Geometry check sheet. Reference: drawing and pictorial views, mm from the part's lowest x, y, z. A direction names the side the tool comes from. Give positions to 0.01 mm unless a question says otherwise; leave off trailing zeros. Write each loop counter-clockwise with the first axis right and the second up, starting at its lowest first coordinate (ties: lowest second). Pieces come first, ordered by that corner, then holes. Notation, with made-up numbers: M 82,47.25 L 104,47.25 A20 cw 104,83.25 Z; hole C -13.5,10 d4. An arc over 180 degrees is marked long. Answer as a JSON object with one key per item and string values.
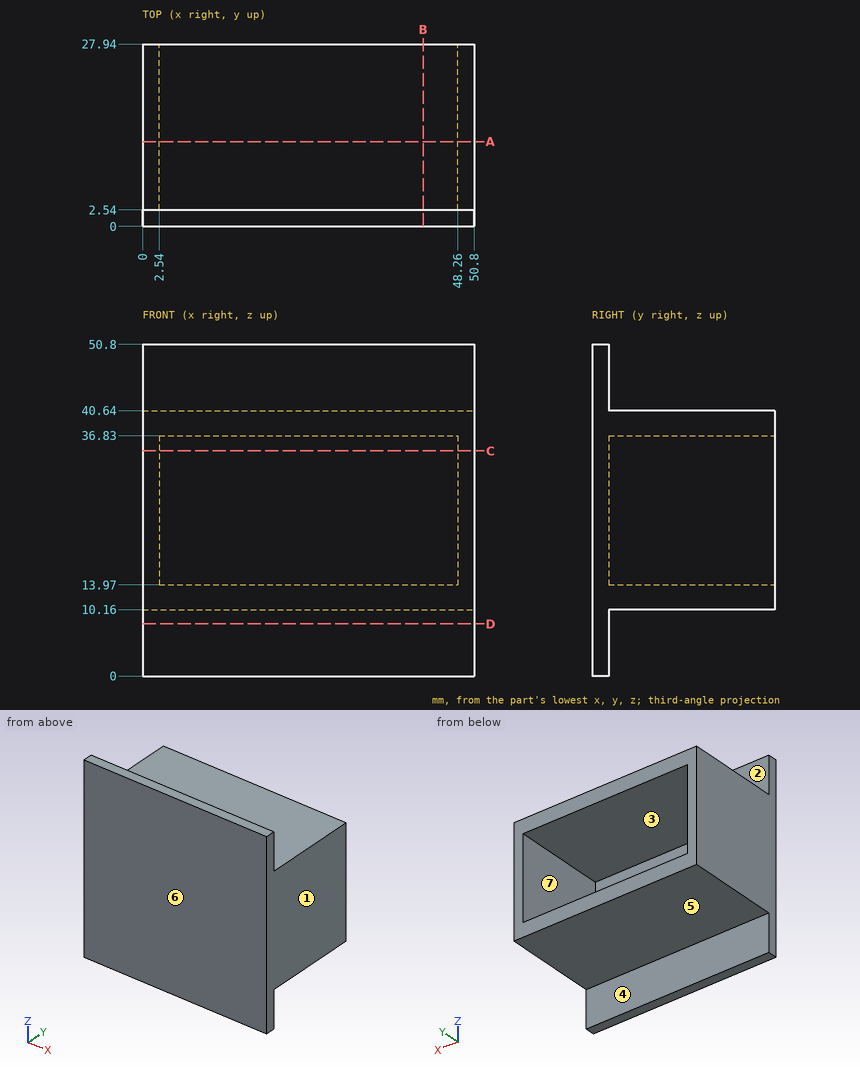
1) Release check for a two-part mould opening along Z. For the marked faces 5, 6 and 7 record: pulls with the +Z half, pulls with the -Z half, needs draft (parallel to the pull), parting line crosses it, or undercut.
Completed:
{"face 5": "pulls with the -Z half", "face 6": "needs draft", "face 7": "undercut"}
2) Section check B-B on x = 43. Record the boundary of the cut face in (y, z).
Completed:
{"outline": "M 0,0 L 2.54,0 L 2.54,10.16 L 27.94,10.16 L 27.94,13.97 L 2.54,13.97 L 2.54,36.83 L 27.94,36.83 L 27.94,40.64 L 2.54,40.64 L 2.54,50.8 L 0,50.8 Z"}
3) Section check C-C on z = 34.5. Record the boundary of the cut face in (x, y).
Completed:
{"outline": "M 0,0 L 50.8,0 L 50.8,27.94 L 48.26,27.94 L 48.26,2.54 L 2.54,2.54 L 2.54,27.94 L 0,27.94 Z"}
4) Section check A-A on y = 13. Record the boundary of the cut face in (x, z), and give its area (3 significant figures).
Completed:
{"outline": "M 0,10.16 L 50.8,10.16 L 50.8,40.64 L 0,40.64 Z; hole M 2.54,13.97 L 48.26,13.97 L 48.26,36.83 L 2.54,36.83 Z", "area": "503 mm2"}
5) Thickness scan on L1, parallel to X at y = 25.25, z = 18; L2, parallel to Z at x = 23, y = 25.25; L3, parallel to Y at x = 28, z = 4. Record the ranges inside material, lowest first.
Completed:
{"L1": "x = 0 to 2.54, 48.26 to 50.8", "L2": "z = 10.16 to 13.97, 36.83 to 40.64", "L3": "y = 0 to 2.54"}
6) Go/stop test with flat-tipped pins: pin 1 (3 mm diameter, centred on x = 15.5, y = 23, fed in from -Z); pin 2 (5 mm diameter, centred on x = 14.5, z = 7.5, fed in from +Y); pin 3 (3 mm diameter, centred on x = 38, y = 17, fed in from +Z). Record where each tip stops, or that it passes through.
Completed:
{"pin 1": "stops at z = 10.16", "pin 2": "stops at y = 2.54", "pin 3": "stops at z = 40.64"}
7) Access from +Z, -Z, +X, -X, +Y, -Y to the whole of each face (thin tool, end or side, straight path). Record for the marked faces 1, 2, 3 and 4.
Completed:
{"face 1": "+Z, -Z, +X, +Y, -Y", "face 2": "+Z, +X, -X, +Y", "face 3": "+Y", "face 4": "-Z, +X, -X, +Y"}
8) Section check D-D on z = 8. Record the boundary of the cut face in (x, y).
Completed:
{"outline": "M 0,0 L 50.8,0 L 50.8,2.54 L 0,2.54 Z"}
